Read the model definition and answer for the solid it produces. Units are mm, in the model's axes. Give positions to 0.01 mm unless a question says otherwise; leave off trailing zeros. Loops run counter-clockwise (first coordinate to the right, second up) from the corner with the lowest first, then second, coordinate; pieces in that order, holes last. Notation, with made-up numbers: (23.25, 28.25) - (57.25, 28.25) arc R9 ccw to (57.25, 33.25) - close; hole circle Ø6 at (70, -20.5). An arc over 180 degrees is marked (long way). Put each result on its own line as item: value. Start each with the question number.
1. Consider L1, parallel to Y at x = 19.5, z = 3.5; L2, parallel to X at y = 63.5, z = 7.25 (3 decimals); L3, parallel to X at y = 76, z = 11.5. Determine where each line is inside the solid, lowest interval first. Write a range as from..to.
2. For a pull along Y with two mould halves and no side action, classify faces 1 (the cylindrical face through (10.959, 9.586, 12.325)), 2 (the flat face through (3, 44, 0)), 3 (the cylindrical face through (-15.875, 63.528, 12.325)), 4 (the flat face through (12.687, 37.203, 12.325)) as released by +Y, released by -Y, zero draft, split by the parting line, or undercut.
3. A cutting plane is placed at C-C, the plane y = 56. Determine the outline of the cut face in (x, z).
4. A cutting plane is placed at B-B, the plane x = 37. Determine the outline of the cut face in (y, z), plus the area to 3 significant figures.
5. Given pin 1 Ø2 at (y, z) = (56, 16.5) entering from -X; pin 2 Ø5 at (x, z) = (29, 12) entering from +Y; pin 3 Ø4 at (y, z) = (45.5, 22.5) entering from -X, each flat-ended and moving along its own axis, determine where each tip first touches the part or whether it passes through.
```python
from build123d import *

# Parameters (mm, degrees)
F1_DEPTH = 25


with BuildPart() as f1:
    # F0 (on Top) → F1 (new body)
    with BuildSketch(Plane.XY):
        with BuildLine():
            ThreePointArc((0, -7.9375), (5.6126600757, -5.6126600757), (7.9375, 0))
            ThreePointArc((7.9375, 0), (-0.4970693683, 7.9219207452), (-7.8752441368, -0.9921875))
            ThreePointArc((-7.8752441368, -0.9921875), (-5.2501627579, -5.953125), (0, -7.9375))
        make_face()
        with BuildLine():
            ThreePointArc((44.45, 7.9375), (36.5125, 0), (44.45, -7.9375))
            ThreePointArc((44.45, -7.9375), (50.0626600757, -5.6126600757), (52.3875, 0))
            ThreePointArc((52.3875, 0), (50.0626600757, 5.6126600757), (44.45, 7.9375))
        make_face()
        with BuildLine():
            ThreePointArc((-15.7504882737, 65.484375), (-15.875, 63.5), (-15.7504882737, 61.515625))
            ThreePointArc((-15.7504882737, 61.515625), (0, 47.625), (15.7504882737, 61.515625))
            ThreePointArc((15.7504882737, 61.515625), (15.8438414904, 62.5058612634), (15.875, 63.5))
            ThreePointArc((15.875, 63.5), (15.8438414904, 64.4941387366), (15.7504882737, 65.484375))
            ThreePointArc((15.7504882737, 65.484375), (0, 79.375), (-15.7504882737, 65.484375))
        make_face()
        with BuildLine():
            ThreePointArc((-7.8752441368, -0.9921875), (-0.4970693683, 7.9219207452), (7.9375, 0))
            ThreePointArc((7.9375, 0), (5.6126600757, -5.6126600757), (0, -7.9375))
            Line((0, -7.9375), (44.45, -7.9375))
            ThreePointArc((44.45, -7.9375), (36.5125, 0), (44.45, 7.9375))
            Line((44.45, 7.9375), (14.6697461087, 7.9375))
            ThreePointArc((14.6697461087, 7.9375), (10.9197461087, 9.6303108612), (9.7089624004, 13.5625))
            Line((9.7089624004, 13.5625), (15.7504882737, 61.515625))
            ThreePointArc((15.7504882737, 61.515625), (0, 47.625), (-15.7504882737, 61.515625))
            Line((-15.7504882737, 61.515625), (-7.8752441368, -0.9921875))
        make_face()
        with BuildLine():
            Line((-9.4502929642, 115.490625), (-15.7504882737, 65.484375))
            ThreePointArc((-15.7504882737, 65.484375), (0, 79.375), (15.7504882737, 65.484375))
            Line((15.7504882737, 65.484375), (9.4502929642, 115.490625))
            ThreePointArc((9.4502929642, 115.490625), (9.5063048942, 114.896483242), (9.525, 114.3))
            ThreePointArc((9.525, 114.3), (-0.596483242, 104.7936951058), (-9.4502929642, 115.490625))
        make_face()
        with BuildLine():
            ThreePointArc((9.4502929642, 115.490625), (0, 123.825), (-9.4502929642, 115.490625))
            ThreePointArc((-9.4502929642, 115.490625), (-0.596483242, 104.7936951058), (9.525, 114.3))
            ThreePointArc((9.525, 114.3), (9.5063048942, 114.896483242), (9.4502929642, 115.490625))
        make_face()
    extrude(amount=F1_DEPTH)


solid = f1.part
```
Return value:
1. L1: y = -7.94..7.94
1. L2: x = -15.875..15.875
1. L3: x = -14.43..14.43
2. face 1: undercut
2. face 2: zero draft
2. face 3: split by the parting line
2. face 4: undercut
3. outline: (-15.06, 0) - (15.06, 0) - (15.06, 25) - (-15.06, 25) - close
4. outline: (-7.94, 0) - (7.94, 0) - (7.94, 25) - (-7.94, 25) - close
4. area: 397 mm2
5. pin 1: stops at x = -15.18
5. pin 2: stops at y = 7.94
5. pin 3: stops at x = -13.98
